The model under review builds one solid part; all positions refer to its coordinate system, in mm. A direction names the side the tool comes from. Give positions to 0.01 mm unless a question says otherwise; leave off trailing zeros. Loops run counter-clockwise (first coordinate to the right, second up) from the corner with the lowest first, then second, coordinate; pieces in that order, holes last. Notation, with made-up numbers: M -4,40.5 L 36,40.5 A14 cw 36,58.5 Z; hole C 79.5,-27 d3. An arc over 180 degrees is marked long. One line per item, written item: value. Start each with the question number.
Q1. For pin 1 (1 mm diameter, centred on y = 4.5, z = -20.5, fed in from +X); pin 2 (1 mm diameter, centred on y = 2.5, z = -19.5, fed in from -X); pin 3 (1.1 mm diameter, centred on x = -50.5, y = 4.5, fed in from -Z); pin 4 (10 mm diameter, centred on x = -87, z = -10, fed in from -Y), all flat-tipped, find the tip position at first contact; note any pin that passes through.
Q2. Mouldability with a two-part tool opening along Z and no side actions: class faces 1 (the face through (-70.403, 2.958, 16.478)), 2 (the face through (-49, 3, -0.721)), 3 (the face through (-72.685, 3, -26)) as released by +Z, released by -Z, zero draft, split by the parting line, or undercut.
Q3. We need section C-C on z = -21. Write out the cut boundary in (x, y), plus the area to 3 significant figures.
Q4. To check wall thickness, follow line 1 along Z through (x, y) = (-62.5, 4.5); line 2 along X through (y, z) = (4.35, -24.5); line 3 along Z through (x, y) = (-63, 5.15). State the ranges of each line that lie inside material, in increasing order. Write a range as from..to.
Q5. For faces 4 (the face through (-51.011, 3, 1)), 5 (the face through (-79.544, 3.042, -37.612)), 6 (the face through (-82.76, 2.96, 12.46)), list the 3-axis set-ups (+Z, -Z, +X, -X, +Y, -Y) from which the entire face can be reached by the end or side of a thin tool; tool diameter is ignored.
Q6. We need section A-A on x = -71.5. Write out the cut boundary in (y, z), plus the area to 3 significant figures.
Q7. We need section D-D on x = -91.5. Write out the cut boundary in (y, z), plus the area to 3 significant figures.
Q8. We need section B-B on y = 2.1. Give the number of separate pieces and of enclosed holes in the cut face, plus the area to 3 significant figures.
```python
from build123d import *

# Parameters (mm, degrees)
SKETCH1_R           = 2.3
BOSS_EXTRUDE1_DEPTH = 6
FILLET1_R           = 4


with BuildPart() as part:
    # Sketch1 → Boss-Extrude1 (new body)
    with BuildSketch(Plane(origin=(0, 0, 0), x_dir=(1, 0, 0), z_dir=(0, 1, 0))):
        Polygon((-80.684780516, 38.81470852), (-80.684780516, 8.81470852), (-52.494001892, -1.44589578), (-107.0151375, -21.289966279), (-104.278976354, -28.807507246), (-29.103566691, -1.44589578), (-72.684780516, 14.416368826), (-72.684780516, 38.81470852), align=None)
        with Locations(Location((-76.684780516, 33.843739542, 0), (0, 0, 270))):
            Circle(SKETCH1_R, mode=Mode.SUBTRACT)
        Polygon((-51.010936087, -0.6288713), (-51.010936087, -2.3288713), (-49.660936087, -2.3288713), (-49.660936087, -3.6788713), (-47.960936087, -3.6788713), (-47.960936087, -2.3288713), (-46.610936087, -2.3288713), (-46.610936087, -0.6288713), (-47.960936087, -0.6288713), (-47.960936087, 0.7211287), (-49.660936087, 0.7211287), (-49.660936087, -0.6288713), align=None, mode=Mode.SUBTRACT)
    extrude(amount=BOSS_EXTRUDE1_DEPTH)

    # Fillet1
    fillet1_edges = [part.edges().sort_by_distance(p)[0] for p in [
        (-72.684780516, 3, -14.416368826),
        (-80.684780516, 3, -8.81470852),
        (-104.278976354, 3, 28.807507246),
        (-107.0151375, 3, 21.289966279),
        (-52.494001892, 3, 1.44589578),
        (-29.103566691, 3, 1.44589578),
        (-72.684780516, 3, -38.81470852),
        (-80.684780516, 3, -38.81470852),
    ]]
    fillet(fillet1_edges, radius=FILLET1_R - 0.0001)  # a hair under: the kernel refuses the full size


solid = part.part
```
Solved:
1. pin 1: x = -72.68
1. pin 2: x = -80.68
1. pin 3: z = -6.54
1. pin 4: through
2. face 1: released by +Z
2. face 2: undercut
2. face 3: zero draft
3. outline: M -80.68,0 L -72.68,0 L -72.68,6 L -80.68,6 Z
3. area: 48.0 mm2
4. line 1: -10.71..-2.18, 5.07..13.6
4. line 2: -80.68..-72.68
4. line 3: -10.89..-2.38, 5.27..13.78
5. face 4: +Y, -Y
5. face 5: -Z, -X, +Y, -Y
5. face 6: -X, +Y, -Y
6. outline: M 0,-14.38 L 6,-14.38 L 6,-5.47 L 0,-5.47 Z; M 0,8.36 L 6,8.36 L 6,16.88 L 0,16.88 Z
6. area: 105 mm2
7. outline: M 0,15.64 L 6,15.64 L 6,24.16 L 0,24.16 Z
7. area: 51.1 mm2
8. separate pieces: 1
8. enclosed holes: 2
8. area: 1,030 mm2
